from build123d import *

# Parameters (mm, degrees)
SKETCH1_W                            = 112.65
SKETCH1_H                            = 90
BOSS_EXTRUDE1_DEPTH                  = 3.175
M4_CLEARANCE_HOLE1_D                 = 4.5
MIRROR1_AT_THE_SECOND_PLANE_COPY_1_D = 4.5


with BuildPart() as part:
    # Sketch1 → Boss-Extrude1 (new body)
    with BuildSketch(Plane.XY):
        Rectangle(SKETCH1_W, SKETCH1_H)
    extrude(amount=BOSS_EXTRUDE1_DEPTH)

    # M4 Clearance Hole1 (through all)
    with Locations(Plane.XY.offset(3.175)):
        with Locations((-48.15, -40)):
            m4_clearance_hole1 = Hole(M4_CLEARANCE_HOLE1_D / 2)

    # Mirror1: M4 Clearance Hole1 across plane
    add(m4_clearance_hole1.mirror(Plane(origin=(0, 0, 0), x_dir=(0, 0, 1), z_dir=(1, 0, 0))), mode=Mode.SUBTRACT)

    # Mirror1 at the second plane: M4 Clearance Hole1 across plane
    add(m4_clearance_hole1.mirror(Plane.ZX), mode=Mode.SUBTRACT)

    # Mirror1 at the second plane copy 1 (through all)
    with Locations(Plane(origin=(0, 0, 3.175), x_dir=(-1, 0, 0), z_dir=(0, 0, 1))):
        with Locations((-48.15, -40)):
            Hole(MIRROR1_AT_THE_SECOND_PLANE_COPY_1_D / 2)


solid = part.part
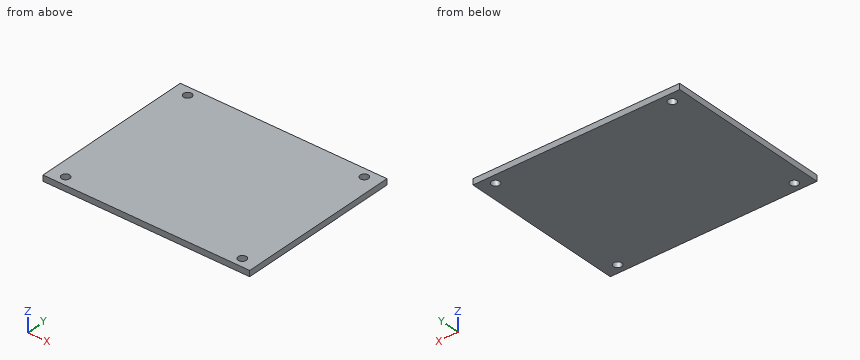
CAD build for the part. Positions are in the model's coordinates, mm. Round coordinates to 2 decimals unless told otherwise and drop trailing zeros. Loops run counter-clockwise (first coordinate to the right, second up) from the corner with the lowest first, then second, coordinate; pieces in that order, holes last.
(1) Wall check: line 1 along Y through (x, z) = (-48.15, 1.45); line 2 along X through (y, z) = (-38, 0.4) (3 decimals); line 3 along Y through (x, z) = (49.5, 0.35). Give the ranges that are in metal, low to high.
(2) Cut at A-A (x = 48.15). Give the cut face in (y, z) (3 decimals).
(3) Cut at B-B (y = -40). Give the cut face in (x, z) (3 decimals), plus the area to 3 significant figures.
Findings below:
1. line 1: y = -45 to -42.25, -37.75 to 37.75, 42.25 to 45
1. line 2: x = -56.325 to -49.181, -47.119 to 47.119, 49.181 to 56.325
1. line 3: y = -45 to -41.8, -38.2 to 38.2, 41.8 to 45
2. outline: (-45, 0) - (-42.25, 0) - (-42.25, 3.175) - (-45, 3.175) - close; (-37.75, 0) - (37.75, 0) - (37.75, 3.175) - (-37.75, 3.175) - close; (42.25, 0) - (45, 0) - (45, 3.175) - (42.25, 3.175) - close
3. outline: (-56.325, 0) - (-50.4, 0) - (-50.4, 3.175) - (-56.325, 3.175) - close; (-45.9, 0) - (45.9, 0) - (45.9, 3.175) - (-45.9, 3.175) - close; (50.4, 0) - (56.325, 0) - (56.325, 3.175) - (50.4, 3.175) - close
3. area: 329 mm2
